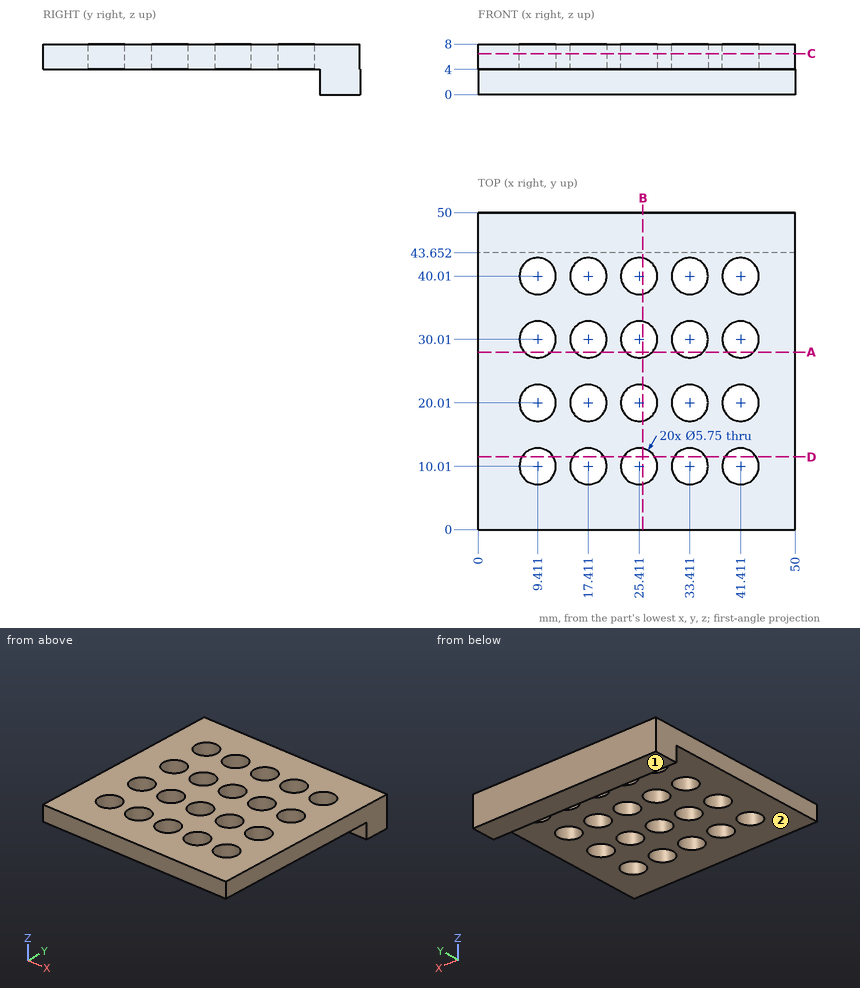
The drawing under review shows one solid part. Ordinate dimensions are in mm from its lowest x, y, z. A direction names the side the tool comes from. Coordinates: 2 decimals unless noted, no trailing zeros. Write each loop counter-clockwise with the first axis right and the second up, starting at its lowest first coordinate (ties: lowest second). Pieces come first, ordered by that corner, then holes.
1) Add section A-A (y = 28). Write out the cut boundary in (x, z) (1 decimal).
2) To check wall thickness, follow L1, parallel to Y at x = 42.5, z = 4.5; L2, parallel to Y at x = 17, z = 7.75 (1 decimal); L3, parallel to X at y = 32, z = 4.5 (1 decimal). State the ranges of each line that lie inside material, in increasing order.
3) Add section C-C (z = 6.5). State how many separate pieces and enclosed holes the cut face has, plus the area to 3 significant figures.
4) Add section B-B (x = 26). Write out the cut boundary in (y, z), plus the area to 3 significant figures.
5) Add section D-D (y = 11.5). Write out the cut boundary in (x, z).
6) Machinability: for the marked faces 1 and 2, which of the approach directions +Z, -Z, +X, -X, +Y, -Y give a long, thin tool a straight path to every point of the face, cutting with its end or side? Answer none if there is none.
7) Insertion check: pin 1 (13 mm diameter, centred on x = 12.5, y = 24.5, fed in from -Z). The pin has a flat end and moves straight along its axis. Give the tip position at first contact, or say it passes through.
Check result:
1. outline: (0, 4) - (7.4, 4) - (7.4, 8) - (0, 8) - close; (11.5, 4) - (15.4, 4) - (15.4, 8) - (11.5, 8) - close; (19.5, 4) - (23.4, 4) - (23.4, 8) - (19.5, 8) - close; (27.5, 4) - (31.4, 4) - (31.4, 8) - (27.5, 8) - close; (35.5, 4) - (39.4, 4) - (39.4, 8) - (35.5, 8) - close; (43.5, 4) - (50, 4) - (50, 8) - (43.5, 8) - close
2. L1: y = 0 to 7.35, 12.67 to 17.35, 22.67 to 27.35, 32.67 to 37.35, 42.67 to 50
2. L2: y = 0 to 7.2, 12.9 to 17.2, 22.9 to 27.2, 32.9 to 37.2, 42.9 to 50
2. L3: x = 0 to 7.3, 11.5 to 15.3, 19.5 to 23.3, 27.5 to 31.3, 35.5 to 39.3, 43.5 to 50
3. separate pieces: 1
3. enclosed holes: 20
3. area: 1,980 mm2
4. outline: (0, 4) - (7.2, 4) - (7.2, 8) - (0, 8) - close; (12.82, 4) - (17.2, 4) - (17.2, 8) - (12.82, 8) - close; (22.82, 4) - (27.2, 4) - (27.2, 8) - (22.82, 8) - close; (32.82, 4) - (37.2, 4) - (37.2, 8) - (32.82, 8) - close; (42.82, 4) - (43.65, 4) - (43.65, 0) - (50, 0) - (50, 8) - (42.82, 8) - close
4. area: 135 mm2
5. outline: (0, 4) - (6.95, 4) - (6.95, 8) - (0, 8) - close; (11.87, 4) - (14.95, 4) - (14.95, 8) - (11.87, 8) - close; (19.87, 4) - (22.95, 4) - (22.95, 8) - (19.87, 8) - close; (27.87, 4) - (30.95, 4) - (30.95, 8) - (27.87, 8) - close; (35.87, 4) - (38.95, 4) - (38.95, 8) - (35.87, 8) - close; (43.87, 4) - (50, 4) - (50, 8) - (43.87, 8) - close
6. face 1: -Z, +X, -X, +Y, -Y
6. face 2: -Z, +X, -X, -Y
7. pin 1: stops at z = 4
